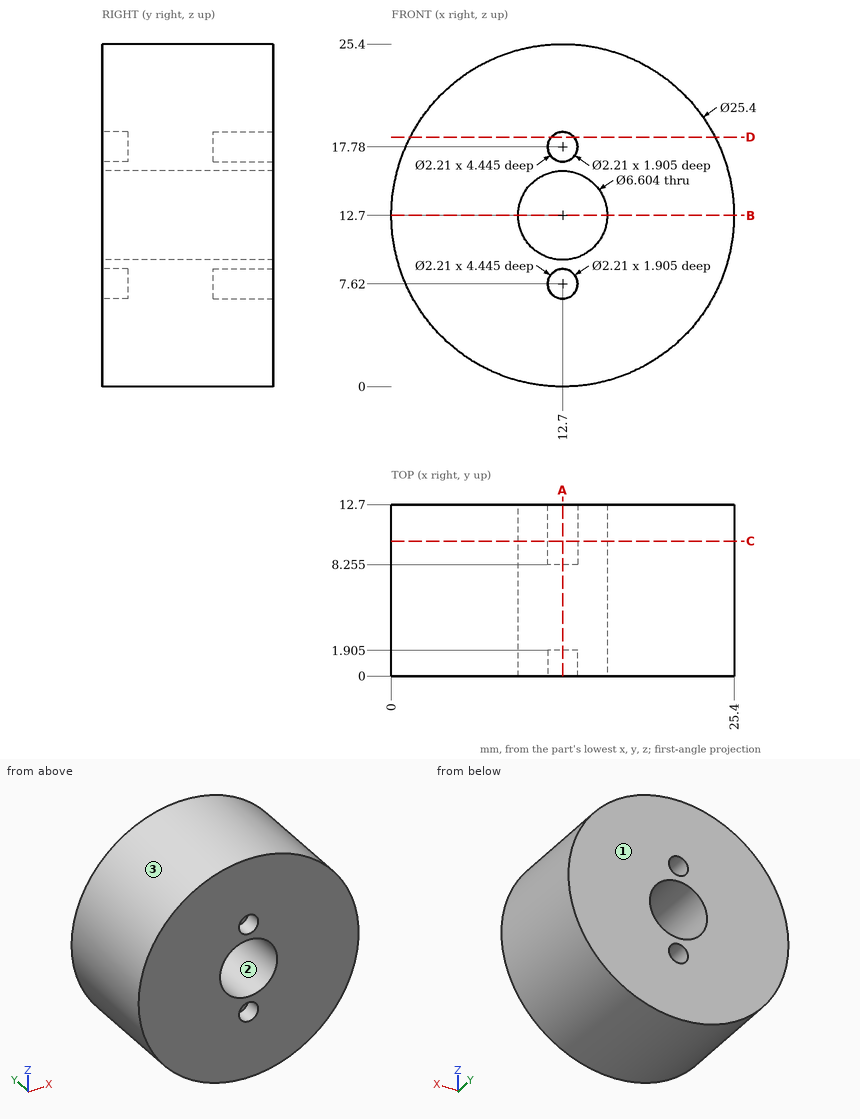
The drawing under review shows one solid part. Ordinate dimensions are in mm from its lowest x, y, z. Round coordinates to 2 decimals unless told otherwise and drop trailing zeros. Loops run counter-clockwise (first coordinate to the right, second up) from the corner with the lowest first, then second, coordinate; pieces in that order, holes last. Notation, with made-up numbers: (22, -22) - (37, -22) arc R17 ccw to (37, -1) - close; hole circle Ø9 at (37, -4.75). An arc over 180 degrees is marked (long way). Use a Markdown table: item, result. Add a question column.
Q1. For probe 1 along Z at (x, y) = (12.7, 1.15) (1 decimal); probe 2 along Z at (x, y) = (12.7, 4.75); probe 3 along X at (y, z) = (0.7, 17.78) (1 decimal), list the stretches that pass through material, from the lowest coordinate up.
Q2. The part is to be moulded in two halves that separate along X. For the marked faces 1, 2 and 3, say which applies: pulls with the +X half, pulls with the -X half, needs draft (parallel to the pull), parting line crosses it, or undercut.
Q3. Insertion check: pin 1 Ø1.8 at (x, z) = (12.7, 17.78) entering from -Y (3 decimals); pin 2 Ø3 at (x, y) = (22, 1.5) entering from -Z; pin 3 Ø5 at (x, y) = (6, 7.5) entering from -Z (1 decimal). Each pin has a flat end and moves straight along its axis. Give the tip position at first contact, or say it passes through.
Q4. Add section C-C (y = 10). State the section outline as (x, z) points (1 decimal), plus the area to 3 significant figures.
Q5. Add section B-B (z = 12.7). State the section outline as (x, y) points, plus the area to 3 significant figures.
Q6. Add section D-D (z = 18.5). State the section outline as (x, y) points (1 decimal).
Q7. Add section A-A (x = 12.7). State the section outline as (y, z) points (1 decimal), plus the area to 3 significant figures.
Worked answers:
| question | item | result |
|---|---|---|
| 1 | probe 1 | 0 to 6.5, 8.7 to 9.4, 16 to 16.7, 18.9 to 25.4 |
| 1 | probe 2 | 0 to 9.4, 16 to 25.4 |
| 1 | probe 3 | 1.1 to 11.6, 13.8 to 24.3 |
| 2 | face 1 | needs draft |
| 2 | face 2 | undercut |
| 2 | face 3 | parting line crosses it |
| 3 | pin 1 | y = 1.905 |
| 3 | pin 2 | z = 2.68 |
| 3 | pin 3 | z = 0.7 |
| 4 | outline | circle Ø25.4 at (12.7, 12.7); hole circle Ø6.6 at (12.7, 12.7); hole circle Ø2.2 at (12.7, 7.6); hole circle Ø2.2 at (12.7, 17.8) |
| 4 | area | 465 mm² |
| 5 | outline | (0, 0) - (9.4, 0) - (9.4, 12.7) - (0, 12.7) - close; (16, 0) - (25.4, 0) - (25.4, 12.7) - (16, 12.7) - close |
| 5 | area | 239 mm² |
| 6 | outline | (1.4, 0) - (11.9, 0) - (11.9, 1.9) - (13.5, 1.9) - (13.5, 0) - (24, 0) - (24, 12.7) - (13.5, 12.7) - (13.5, 8.3) - (11.9, 8.3) - (11.9, 12.7) - (1.4, 12.7) - close |
| 7 | outline | (0, 0) - (12.7, 0) - (12.7, 6.5) - (8.3, 6.5) - (8.3, 8.7) - (12.7, 8.7) - (12.7, 9.4) - (0, 9.4) - (0, 8.7) - (1.9, 8.7) - (1.9, 6.5) - (0, 6.5) - close; (0, 16) - (12.7, 16) - (12.7, 16.7) - (8.3, 16.7) - (8.3, 18.9) - (12.7, 18.9) - (12.7, 25.4) - (0, 25.4) - (0, 18.9) - (1.9, 18.9) - (1.9, 16.7) - (0, 16.7) - close |
| 7 | area | 211 mm² |
